Model file for the job. Use its own axes, mm. A direction names the side the tool comes from. Coordinates: 2 decimals unless noted, no trailing zeros. Order: outer loops, then holes, each group sorted by start corner. A loop starts at its lowest first (then second) coordinate and runs counter-clockwise, first axis right, second up.
from build123d import *

# Parameters (mm, degrees)
SKETCH1_R           = 10
SKETCH1_R_2         = 1.5
BOSS_EXTRUDE1_DEPTH = 2
SKETCH2_R           = 4
SKETCH2_R_2         = 2
BOSS_EXTRUDE2_DEPTH = 3


with BuildPart() as part:
    # Sketch1 → Boss-Extrude1 (new body)
    with BuildSketch(Plane(origin=(0, 0, 0), x_dir=(1, 0, 0), z_dir=(0, 1, 0))):
        Circle(SKETCH1_R)
        with Locations((0, 7)):
            Circle(SKETCH1_R_2, mode=Mode.SUBTRACT)
        with Locations((7, 0)):
            Circle(SKETCH1_R_2, mode=Mode.SUBTRACT)
        with Locations((0, -7)):
            Circle(SKETCH1_R_2, mode=Mode.SUBTRACT)
        with Locations((-7, 0)):
            Circle(SKETCH1_R_2, mode=Mode.SUBTRACT)
    extrude(amount=BOSS_EXTRUDE1_DEPTH)

    # Sketch2 → Boss-Extrude2 (add)
    with BuildSketch(Plane.XZ):
        Circle(SKETCH2_R)
        Circle(SKETCH2_R_2, mode=Mode.SUBTRACT)
    extrude(amount=BOSS_EXTRUDE2_DEPTH)


solid = part.part
Q1. Which spindle directions (+Z, -Z, +X, -X, +Y, -Y) get a long thin tool onto all of the face, cutting with end or side? Do faces 1 (the face through (-0.1, 0, 4.3)), 2 (the face through (-2.17, 0.99, 9.76)). Say none if no direction does.
Established:
face 1: -Y
face 2: +Y, -Y
Q2. Probe line 1 (X direction, y = 1.1, z = 0); line 2 (Y direction, x = -4, z = 3.5). List the from-to ranges inside material, lowest first.
Established:
line 1: x = -10 to -8.5, -5.5 to 5.5, 8.5 to 10
line 2: y = 0 to 2
Q3. Cut at A-A, the plane x = 0. List the corners of the cut face in (y, z), plus the area to 3 significant figures.
Established:
outline: (-3, -4) - (0, -4) - (0, -5.5) - (2, -5.5) - (2, 5.5) - (0, 5.5) - (0, 4) - (-3, 4) - (-3, 2) - (0, 2) - (0, -2) - (-3, -2) - close; (0, -10) - (2, -10) - (2, -8.5) - (0, -8.5) - close; (0, 8.5) - (2, 8.5) - (2, 10) - (0, 10) - close
area: 40.0 mm2
Q4. Cut at C-C, the plane x = -7. List the corners of the cut face in (y, z).
Established:
outline: (0, -7.14) - (2, -7.14) - (2, -1.5) - (0, -1.5) - close; (0, 1.5) - (2, 1.5) - (2, 7.14) - (0, 7.14) - close
Q5. Cut at B-B, the plane z = 7. List the corners of the cut face in (x, y).
Established:
outline: (-7.14, 0) - (-1.5, 0) - (-1.5, 2) - (-7.14, 2) - close; (1.5, 0) - (7.14, 0) - (7.14, 2) - (1.5, 2) - close
Q6. Cut at D-D, the plane z = -1.25. List the corners of the cut face in (x, y), plus the area to 3 significant figures.
Established:
outline: (-9.92, 0) - (-7.83, 0) - (-7.83, 2) - (-9.92, 2) - close; (-6.17, 0) - (-3.8, 0) - (-3.8, -3) - (-1.56, -3) - (-1.56, 0) - (1.56, 0) - (1.56, -3) - (3.8, -3) - (3.8, 0) - (6.17, 0) - (6.17, 2) - (-6.17, 2) - close; (7.83, 0) - (9.92, 0) - (9.92, 2) - (7.83, 2) - close
area: 46.5 mm2
Q7. Drop flat-ended pins along their axis: P1, Ø2, axis at x = 0.5, z = -0.5, coming from the -Y side; P2, Ø6, axis at x = -4, z = -1, coming from the -Y side; P3, Ø1.5, axis at x = -1.5, y = -1, coming from the -Z side; P4, Ø3, axis at x = -3.5, y = -0.5, coming from the +Z side. Give the stop position or say it passes through.
Established:
P1: stops at y = 0
P2: stops at y = -3
P3: stops at z = -3.93
P4: stops at z = 9.78
Q8. Mould opens along X. For faces 3 (the face through (0, 2, 0)), 4 (the face through (-0.867, -1.479, -3.905)), 5 (the face through (5.5, 0.99, -0.07)) say: pulls with the +X half, pulls with the -X half, needs draft (parallel to the pull), parting line crosses it, or undercut.
Established:
face 3: needs draft
face 4: parting line crosses it
face 5: undercut
